Geometry: see drawing. Coordinates: mm, zero at the bounding-box minimum. A direction names the side the tool comes from. Round coordinates to 2 decimals unless told otherwise and drop trailing zeros. Order: outer loops, then holes, each group sorted by start corner. A loop starts at its lowest first (then second) coordinate and runs counter-clockwise, first axis right, second up. Notation, with made-up numbers: (-33, 6.5) -> (-19, 6.5) arc R3 ccw to (-19, 10.5) -> close; hole circle Ø11 at (25.5, 12). An arc over 180 degrees is marked (long way). One line per item, written item: value. Start each with the question number.
1) Reachability of the marked faces 1, 2 and 3 from +Z, -Z, +X, -X, +Y, -Y: full face, straight path, thin tool, end or side. Return the list, or none.
2) Section A-A (y = 12.7). Return the cut outline in (x, z) (1 decimal).
3) Pin query (flat end, axial travel): P1, Ø1, axis at y = 29.5, z = 1.5, coming from the -X side (3 decimals); P2, Ø5, axis at x = 12.7, y = 12.7, coming from the +Z side; P3, Ø1, axis at y = 31.5, z = 1.5, coming from the +X side (3 decimals); P4, Ø1, axis at y = 21, z = 2.5, coming from the +X side. Return the tip coordinate at first contact, or that it passes through.
4) Ray query, L1, parallel to Y at x = 12.7, z = 1.3 (1 decimal); L2, parallel to X at y = 29, z = 0.25 (1 decimal); L3, parallel to X at y = 15.5, z = 2.8 (1 decimal). Return the intervals inside material, ascending.
5) Section D-D (y = 35). Return the cut outline in (x, z) (1 decimal).
6) Section B-B (x = 12.7). Return the cut outline in (y, z) (1 decimal).
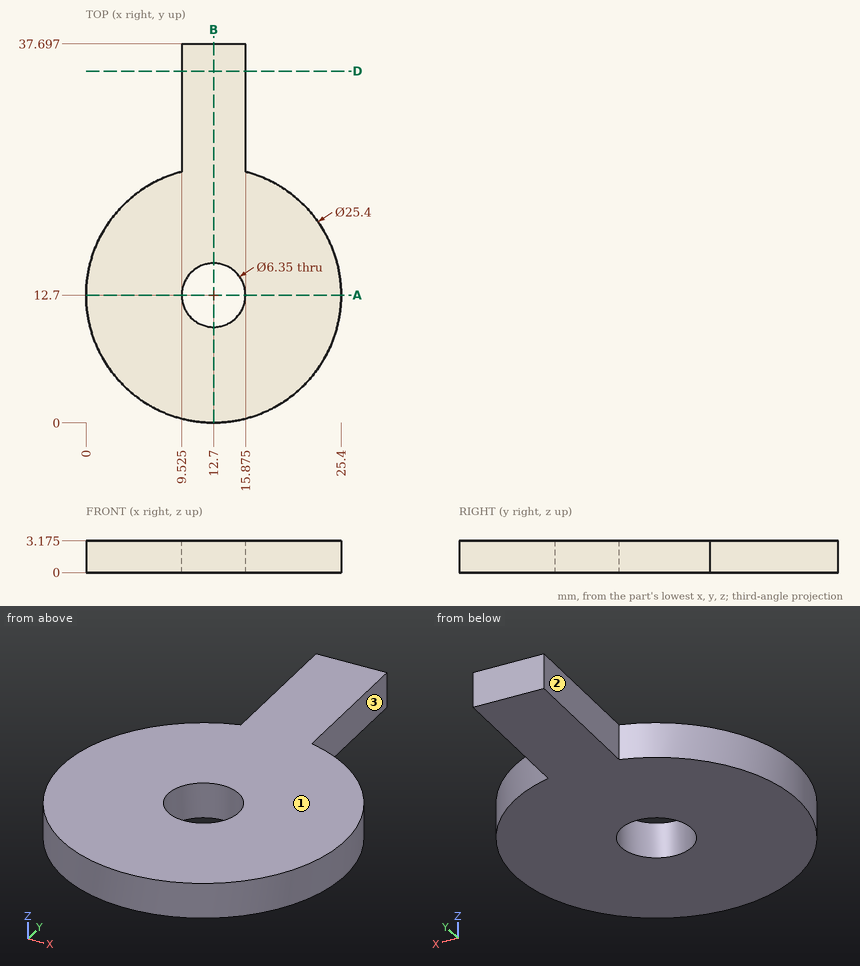
Findings:
1. face 1: +Z, +X, -X, +Y, -Y
1. face 2: +Z, -Z, -X, +Y
1. face 3: +Z, -Z, +X, +Y
2. outline: (0, 0) -> (9.5, 0) -> (9.5, 3.2) -> (0, 3.2) -> close; (15.9, 0) -> (25.4, 0) -> (25.4, 3.2) -> (15.9, 3.2) -> close
3. P1: x = 9.525
3. P2: through
3. P3: x = 15.875
3. P4: x = 22.72
4. L1: 0 to 9.5, 15.9 to 37.7
4. L2: 9.5 to 15.9
4. L3: 0.3 to 11.2, 14.2 to 25.1
5. outline: (9.5, 0) -> (15.9, 0) -> (15.9, 3.2) -> (9.5, 3.2) -> close
6. outline: (0, 0) -> (9.5, 0) -> (9.5, 3.2) -> (0, 3.2) -> close; (15.9, 0) -> (37.7, 0) -> (37.7, 3.2) -> (15.9, 3.2) -> close
